CAD build for the part. Positions are in the model's coordinates, mm. A direction names the side the tool comes from. Coordinates: 2 decimals unless noted, no trailing zeros. Loops run counter-clockwise (first coordinate to the right, second up) from the corner with the lowest first, then second, coordinate; pieces in that order, holes last. Notation, with made-up numbers: M 31.25,-26 L 51.25,-26 A13 ccw 51.25,-19 Z; hole C 53,53 d2. An arc over 180 degrees is marked long. Answer as a JSON object with one key per item and string values. Group by question number.
```python
from build123d import *

# Parameters (mm, degrees)
SKETCH1_W           = 80
SKETCH1_H           = 40
BOSS_EXTRUDE1_DEPTH = 60
SKETCH2_R           = 10
CUT_EXTRUDE1_DEPTH  = 60
SKETCH3_W           = 15
SKETCH3_H           = 30
BOSS_EXTRUDE2_DEPTH = 50


with BuildPart() as part:
    # Sketch1 → Boss-Extrude1 (new body)
    with BuildSketch(Plane(origin=(0, 0, 0), x_dir=(0, 0, -1), z_dir=(1, 0, 0))):
        Rectangle(SKETCH1_W, SKETCH1_H)
    extrude(amount=BOSS_EXTRUDE1_DEPTH)

    # Sketch2 → Cut-Extrude1 (cut)
    with BuildSketch(Plane(origin=(0, 0, 0), x_dir=(0, 0, -1), z_dir=(1, 0, 0))):
        Circle(SKETCH2_R)
    extrude(amount=CUT_EXTRUDE1_DEPTH, mode=Mode.SUBTRACT)

    # Sketch3 → Boss-Extrude2 (add)
    with BuildSketch(Plane(origin=(60, 0, 0), x_dir=(0, 0, -1), z_dir=(1, 0, 0))):
        with Locations((0, 25)):
            Rectangle(SKETCH3_W, SKETCH3_H)
        with Locations((0, -25)):
            Rectangle(SKETCH3_W, SKETCH3_H)
    extrude(amount=BOSS_EXTRUDE2_DEPTH)


solid = part.part
```
Item 1: Drill centre lines: L1, parallel to Y at x = 13, z = 0; L2, parallel to Z at x = 17, y = 0; L3, parallel to X at y = -3.5, z = -12. Where is each one in solid material? Low to high. Write a range as from..to.
Item 2: Slice it at C-C, the plane y = 0. Write the cut outline in (x, z), then the cut area to 3 significant figures.
Item 3: Slice it at A-A, the plane x = 78. Write the cut outline in (y, z).
Item 4: Pin check, flat tips, straight feed: pin 1 (1.5 mm diameter, centred on y = 21, z = 1, fed in from -X); pin 2 (9 mm diameter, centred on x = 80.5, y = -25, fed in from +Z); pin 3 (10 mm diameter, centred on x = 75, y = 6, fed in from -Z); pin 4 (16.5 mm diameter, centred on y = -26.5, z = -3.5, fed in from -X). Stop position of each tip, or through.
Item 5: Tool access for faces 1 (the flat face through (60, 30, 0)), 2 (the flat face through (85, 10, 0)), 3 (the flat face through (85, 25, 7.5)), 4 (the flat face through (60, -30, 0)), 5 (the flat face through (85, 25, -7.5)): list every direction of +Z, -Z, +X, -X, +Y, -Y with a clear straight run to the whole face (end or side of a thin tool).
Item 6: Slice it at D-D, the plane y = -15.5. Write the cut outline in (x, z), then the cut area to 3 significant figures.
Item 7: Slice it at B-B, the plane z = 6. Write the cut outline in (x, y), then the cut area to 3 significant figures.
Item 8: Pull direction Y, two halves, no side cores. Call faces 6 (the flat face through (30, 0, 40)), 7 (the cylindrical face through (29.58, -9.76, 2.17)), 8 (the flat face through (85, -40, 0)), 9 (the flat face through (85, -10, 0)): released by +Y, released by -Y, zero draft, split by the parting line, or undercut.
Computed:
{
 "1": {"L1": "-20..-10, 10..20", "L2": "-40..-10, 10..40", "L3": "0..60"},
 "2": {"outline": "M 0,-40 L 60,-40 L 60,-10 L 0,-10 Z; M 0,10 L 60,10 L 60,40 L 0,40 Z", "area": "3,600 mm2"},
 "3": {"outline": "M -40,-7.5 L -10,-7.5 L -10,7.5 L -40,7.5 Z; M 10,-7.5 L 40,-7.5 L 40,7.5 L 10,7.5 Z"},
 "4": {"pin 1": "x = 60", "pin 2": "z = 7.5", "pin 3": "z = -7.5", "pin 4": "x = 0"},
 "5": {"face 1": "+Z, -Z, -X, +Y", "face 2": "+Z, -Z, +X", "face 3": "+Z, +X, +Y, -Y", "face 4": "+Z, -Z, -X, -Y", "face 5": "-Z, +X, +Y, -Y"},
 "6": {"outline": "M 0,-40 L 60,-40 L 60,-7.5 L 110,-7.5 L 110,7.5 L 60,7.5 L 60,40 L 0,40 Z", "area": "5,550 mm2"},
 "7": {"outline": "M 0,-20 L 60,-20 L 60,-40 L 110,-40 L 110,-10 L 60,-10 L 60,-8 L 0,-8 Z; M 0,8 L 60,8 L 60,10 L 110,10 L 110,40 L 60,40 L 60,20 L 0,20 Z", "area": "4,440 mm2"},
 "8": {"face 6": "zero draft", "face 7": "undercut", "face 8": "released by -Y", "face 9": "undercut"}
}
